```python
from build123d import *

# Parameters (mm, degrees)
BOSS_EXTRUDE1_DEPTH = 2.3114
FILLET1_R           = 12.7
SKETCH2_R           = 2.4257
CUT_EXTRUDE1_DEPTH  = 180.619994906
SKETCH3_R           = 2.4257
CUT_EXTRUDE2_DEPTH  = 180.619994906
SKETCH4_R           = 2.4257
CUT_EXTRUDE3_DEPTH  = 180.619994906
SKETCH5_R           = 2.4257
CUT_EXTRUDE4_DEPTH  = 180.619994906
SKETCH6_R           = 2.4257
CUT_EXTRUDE5_DEPTH  = 180.619994906


with BuildPart() as part:
    # Sketch1 → Boss-Extrude1 (new body)
    with BuildSketch(Plane.XY):
        Polygon((0, 0), (0, -127), (21.3614, -127), (21.3614, -21.3614), (127, -21.3614), (127, 0), align=None)
    extrude(amount=BOSS_EXTRUDE1_DEPTH)

    # Fillet1
    fillet1_edges = [part.edges().sort_by_distance(p)[0] for p in [
        (21.3614, -21.3614, 1.1557),
    ]]
    fillet(fillet1_edges, radius=FILLET1_R)

    # Sketch2 → Cut-Extrude1 (cut, through all)
    with BuildSketch(Plane.XY.offset(2.3114)):
        with Locations((9.525, -104.83088)):
            Circle(SKETCH2_R)
        with Locations((94.5261, -9.525)):
            Circle(SKETCH2_R)
    extrude(amount=-CUT_EXTRUDE1_DEPTH, mode=Mode.SUBTRACT)

    # Sketch3 → Cut-Extrude2 (cut, through all)
    with BuildSketch(Plane.XY.offset(2.3114)):
        with Locations((42.1386, -9.525)):
            Circle(SKETCH3_R)
        with Locations((9.525, -10.3886)):
            Circle(SKETCH3_R)
    extrude(amount=-CUT_EXTRUDE2_DEPTH, mode=Mode.SUBTRACT)

    # Sketch4 → Cut-Extrude3 (cut, through all)
    with BuildSketch(Plane.XY.offset(2.3114)):
        with Locations((9.525, -42.1386)):
            Circle(SKETCH4_R)
    extrude(amount=-CUT_EXTRUDE3_DEPTH, mode=Mode.SUBTRACT)

    # Sketch5 → Cut-Extrude4 (cut, through all)
    with BuildSketch(Plane.XY.offset(2.3114)):
        with Locations((9.525, -57.15)):
            Circle(SKETCH5_R)
    extrude(amount=-CUT_EXTRUDE4_DEPTH, mode=Mode.SUBTRACT)

    # Sketch6 → Cut-Extrude5 (cut, through all)
    with BuildSketch(Plane.XY.offset(2.3114)):
        with Locations((57.15, -9.525)):
            Circle(SKETCH6_R)
    extrude(amount=-CUT_EXTRUDE5_DEPTH, mode=Mode.SUBTRACT)


solid = part.part
```
Verification items for the finished model (mm, model axes). Round coordinates to 2 decimals unless told otherwise and drop trailing zeros. Write each loop counter-clockwise with the first axis right and the second up, starting at its lowest first coordinate (ties: lowest second). Pieces come first, ordered by that corner, then holes. Notation, with made-up numbers: (71.5, 67) - (86.5, 67) arc R20 ccw to (86.5, 92) - close; hole circle Ø9 at (3.25, 84.5). An arc over 180 degrees is marked (long way). Answer as a JSON object with one key per item and string values. Group by question number.
Q1. Mould release check, pull along X, two halves, no side actions. Record for faces 1 (the cylindrical face through (10.644, -12.541, 1.172)), 2 (the cylindrical face through (24.983, -25.18, 1.172)), 3 (the flat face through (34, -20, 0)): released by +X, released by -X, zero draft, split by the parting line, or undercut.
Q2. Go/stop test with a flat-tipped pin: pin 1 Ø1 at (x, z) = (113, 1.5) entering from -Y. Record where the tip stops, or that it passes through.
Q3. Thickness scan on line 1 (Y direction, x = 57.15, z = 0.6); line 2 (Y direction, x = 10, z = 0.8); line 3 (Y direction, x = 115, z = 0.4). Record the ranges inside material, lowest first.
Q4. Section check C-C, the plane z = 1.2. Enter the section's corners in (x, y) (3 decimals), plus the area to 3 significant figures.
Q5. Section check A-A, the plane y = -57.15. Enter the section's corners in (x, z).
Q6. Section check B-B, the plane x = 57.15. Enter the section's corners in (y, z), plus the area to 3 significant figures.
Q7. Section check D-D, the plane x = 76. Enter the section's corners in (y, z).
Found:
{
 "1": {"face 1": "undercut", "face 2": "released by +X", "face 3": "zero draft"},
 "2": {"pin 1": "stops at y = -21.36"},
 "3": {"line 1": "y = -21.36 to -11.95, -7.1 to 0", "line 2": "y = -127 to -107.21, -102.45 to -59.53, -54.77 to -44.52, -39.76 to -12.77, -8.01 to 0", "line 3": "y = -21.36 to 0"},
 "4": {"outline": "(0, -127) - (21.361, -127) - (21.361, -34.061) arc R12.7 cw to (34.061, -21.361) - (127, -21.361) - (127, 0) - (0, 0) - close; hole circle Ø4.851 at (9.525, -104.831); hole circle Ø4.851 at (9.525, -57.15); hole circle Ø4.851 at (9.525, -42.139); hole circle Ø4.851 at (9.525, -10.389); hole circle Ø4.851 at (42.139, -9.525); hole circle Ø4.851 at (57.15, -9.525); hole circle Ø4.851 at (94.526, -9.525)", "area": "4,870 mm^2"},
 "5": {"outline": "(0, 0) - (7.1, 0) - (7.1, 2.31) - (0, 2.31) - close; (11.95, 0) - (21.36, 0) - (21.36, 2.31) - (11.95, 2.31) - close"},
 "6": {"outline": "(-21.36, 0) - (-11.95, 0) - (-11.95, 2.31) - (-21.36, 2.31) - close; (-7.1, 0) - (0, 0) - (0, 2.31) - (-7.1, 2.31) - close", "area": "38.2 mm^2"},
 "7": {"outline": "(-21.36, 0) - (0, 0) - (0, 2.31) - (-21.36, 2.31) - close"}
}
